from build123d import *

# Parameters (mm, degrees)
F0_R     = 42.06875
F0_R_2   = 25.4
F1_DEPTH = 120.65
F2_R     = 8.3312
F3_DEPTH = 63.5
F4_R     = 8.3312
F5_DEPTH = 50.8


with BuildPart() as f1:
    # F0 (on Front) → F1 (new body)
    with BuildSketch(Plane.XZ):
        Circle(F0_R)
        Circle(F0_R_2, mode=Mode.SUBTRACT)
    extrude(amount=-F1_DEPTH)

    # F2 (on Right) → F3 (cut, symmetric)
    with BuildSketch(Plane.YZ):
        with Locations((22.225, 0)):
            Circle(F2_R)
    extrude(amount=F3_DEPTH, both=True, mode=Mode.SUBTRACT)

    # F4 (on Top) → F5 (cut, symmetric)
    with BuildSketch(Plane.XY):
        with Locations((0, 98.425)):
            Circle(F4_R)
    extrude(amount=F5_DEPTH, both=True, mode=Mode.SUBTRACT)


solid = f1.part
Design review of the part built by this model. Coordinates are the model's own, in mm. Round coordinates to 2 decimals unless told otherwise and drop trailing zeros. Write each loop counter-clockwise with the first axis right and the second up, starting at its lowest first coordinate (ties: lowest second). Pieces come first, ordered by that corner, then holes. Notation, with made-up numbers: (25.5, 72.25) - (72.5, 72.25) arc R35 cw to (72.5, 105.25) - close; hole circle Ø6 at (67, -23). An arc over 180 degrees is marked (long way). Return JSON: item names as keys, results as strings. Group by question number.
Item 1: For probe 1 along Y at (x, z) = (29, 0); probe 2 along Z at (x, y) = (0, 35); probe 3 along Y at (x, z) = (0, 34.5), list the stretches that pass through material, from the lowest coordinate up. Write a range as [from, to].
Item 2: The part is to be moulded in two halves that separate along Z. For faces 1 (the face through (11.721, 59.48, -22.534)), 2 (the face through (18.1, 0, -18.1)), 3 (the face through (-32.91, 21.14, 8.26)), 4 (the face through (19.412, 59.48, -37.322)), say which applies: pulls with the +Z half, pulls with the -Z half, needs draft (parallel to the pull), parting line crosses it, or undercut.
Item 3: We need section A-A on x = 0. Write out the cut boundary in (y, z), and give its area (3 significant figures).
Item 4: Insertion check: P1, Ø4, axis at y = 61.5, z = -24, coming from the -X side; P2, Ø10, axis at y = 22.5, z = 11.5, coming from the +X side; P3, Ø13.5, axis at y = 22.225, z = 0, coming from the -X side; P4, Ø1, axis at y = 100.5, z = -8.5, coming from the -X side. Each pin has a flat end and moves straight along its axis. Give the tip position at first contact, or say it passes through.
Item 5: We need section C-C on y = 92. Write out the cut boundary in (x, z).
Item 6: We need section D-D on x = 15. Write out the cut boundary in (y, z), and give its area (3 significant figures).
Item 7: We need section B-B on z = 0. Write out the cut boundary in (x, y).
Model answer:
{
 "1": {"probe 1": "y = [0, 13.89], [30.56, 120.65]", "probe 2": "z = [-42.07, -25.4], [25.4, 42.07]", "probe 3": "y = [0, 90.09], [106.76, 120.65]"},
 "2": {"face 1": "undercut", "face 2": "needs draft", "face 3": "undercut", "face 4": "parting line crosses it"},
 "3": {"outline": "(0, -42.07) - (90.09, -42.07) - (90.09, -25.4) - (0, -25.4) - close; (0, 25.4) - (90.09, 25.4) - (90.09, 42.07) - (0, 42.07) - close; (106.76, -42.07) - (120.65, -42.07) - (120.65, -25.4) - (106.76, -25.4) - close; (106.76, 25.4) - (120.65, 25.4) - (120.65, 42.07) - (106.76, 42.07) - close", "area": "3,470 mm²"},
 "4": {"P1": "stops at x = -35.86", "P2": "stops at x = 41.38", "P3": "passes through", "P4": "stops at x = -41.3"},
 "5": {"outline": "(-5.3, -41.73) - (-5.3, -24.84) arc R25.4 cw to (-5.3, 24.84) - (-5.3, 41.73) arc R42.07 ccw to start; (5.3, -41.73) arc R42.07 ccw to (5.3, 41.73) - (5.3, 24.84) arc R25.4 cw to (5.3, -24.84) - close"},
 "6": {"outline": "(0, -39.3) - (120.65, -39.3) - (120.65, -20.5) - (0, -20.5) - close; (0, 20.5) - (120.65, 20.5) - (120.65, 39.3) - (0, 39.3) - close", "area": "4,540 mm²"},
 "7": {"outline": "(-42.07, 0) - (-25.4, 0) - (-25.4, 13.89) - (-42.07, 13.89) - close; (-42.07, 30.56) - (-25.4, 30.56) - (-25.4, 120.65) - (-42.07, 120.65) - close; (25.4, 0) - (42.07, 0) - (42.07, 13.89) - (25.4, 13.89) - close; (25.4, 30.56) - (42.07, 30.56) - (42.07, 120.65) - (25.4, 120.65) - close"}
}
